Print and shaded views of the part. All mm, measured from the part's lowest x, y and z. Give positions to 0.01 mm unless a question says otherwise; leave off trailing zeros. Loops run counter-clockwise (first coordinate to the right, second up) from the corner with the lowest first, then second, coordinate; pieces in that order, holes last. Notation, with made-up numbers: M 26.5,1 L 76.5,1 A10 cw 76.5,14 Z; hole C -16,-30 d1. An arc over 180 degrees is marked long. Answer as CSV lines item,"result".
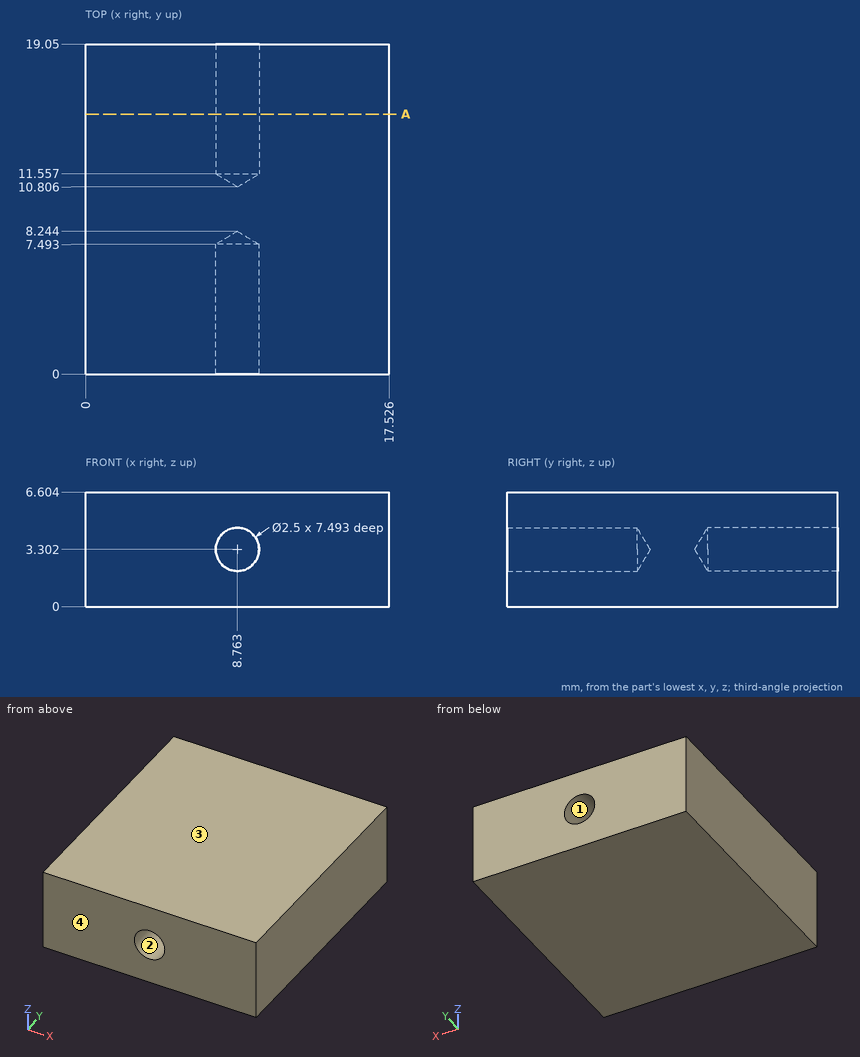
Q1. Pin check, flat tip, straight feed: P1, Ø2, axis at x = 8.763, z = 3.302, coming from the +Y side. Stop position of the tip, or through.
Solution:
P1,"stops at y = 11.41"
Q2. Mould opens along Z. For the marked faces 1, 2, 3 and 4 say: released by +Z, released by -Z, zero draft, split by the parting line, or undercut.
Solution:
face 1,"undercut"
face 2,"undercut"
face 3,"released by +Z"
face 4,"zero draft"
Q3. Cut at A-A (y = 15). Write the cut outline in (x, z), and give its area (3 significant figures).
Solution:
outline,"M 0,0 L 17.53,0 L 17.53,6.6 L 0,6.6 Z; hole C 8.76,3.3 d2.5"
area,"111 mm²"
Q4. Wall check: line 1 (X direction, y = 1.5, z = 2.5); line 2 (Z direction, x = 8, y = 5.5); line 3 (X direction, y = 7.75, z = 3.75). Give the ranges that are in metal, low to high. Write a range as [from, to].
Solution:
line 1,"x = [0, 7.8], [9.72, 17.53]"
line 2,"z = [0, 2.31], [4.29, 6.6]"
line 3,"x = [0, 8.07], [9.45, 17.53]"
